CAD build for the part. Positions are in the model's coordinates, mm. Face numbers are marked on the shaded views. A direction names the side the tool comes from. Coordinates: 2 decimals unless noted, no trailing zeros. Write each loop counter-clockwise with the first axis right and the second up, starting at its lowest first coordinate (ties: lowest second). Pieces come first, ordered by that corner, then holes. Notation, with made-up numbers: M -23,34.5 L 30,34.5 A26 cw 30,48.5 Z; hole C -22.5,1.5 d11. An arc over 180 degrees is marked long. Put each result on its own line as item: value. Start each with the question number.
```python
from build123d import *

# Parameters (mm, degrees)
SALIENTE_EXTRUIR1_DEPTH = 22
CROQUIS2_W              = 34
CROQUIS2_H              = 34
SALIENTE_EXTRUIR2_DEPTH = 7
REDONDEO1_R             = 5
CROQUIS3_R              = 3.5
CORTAR_EXTRUIR1_DEPTH   = 5
CROQUIS4_R              = 2
CORTAR_EXTRUIR2_DEPTH   = 5
CROQUIS5_R              = 3.5
CORTAR_EXTRUIR3_DEPTH   = 5
CROQUIS6_R              = 2
CORTAR_EXTRUIR4_DEPTH   = 5
REDONDEO2_R             = 5


with BuildPart() as part:
    # Croquis1 → Saliente-Extruir1 (new body)
    with BuildSketch(Plane(origin=(0, 0, 0), x_dir=(1, 0, 0), z_dir=(0, 1, 0))):
        Polygon((0, 0), (27, 0), (27, 27), (34, 27), (34, -7), (0, -7), align=None)
    extrude(amount=SALIENTE_EXTRUIR1_DEPTH)

    # Croquis2 → Saliente-Extruir2 (add)
    with BuildSketch(Plane(origin=(0, 0, 0), x_dir=(-1, 0, 0), z_dir=(0, -1, 0))):
        with Locations((-17, 10)):
            Rectangle(CROQUIS2_W, CROQUIS2_H)
    extrude(amount=SALIENTE_EXTRUIR2_DEPTH)

    # Redondeo1
    redondeo1_edges = [part.edges().sort_by_distance(p)[0] for p in [
        (34, 7.5, -27),
        (34, 7.5, 7),
        (0, 7.5, 7),
        (34, -7, -10),
        (17, -7, 7),
    ]]
    fillet(redondeo1_edges, radius=REDONDEO1_R)

    # Croquis3 → Cortar-Extruir1 (cut)
    with BuildSketch(Plane(origin=(34, 0, 0), x_dir=(0, 0, -1), z_dir=(1, 0, 0))):
        with Locations((16, 16)):
            Circle(CROQUIS3_R)
    extrude(amount=-CORTAR_EXTRUIR1_DEPTH, mode=Mode.SUBTRACT)

    # Croquis4 → Cortar-Extruir2 (cut)
    with BuildSketch(Plane(origin=(29, 0, 0), x_dir=(0, 0, -1), z_dir=(1, 0, 0))):
        with Locations((16, 16)):
            Circle(CROQUIS4_R)
    extrude(amount=-CORTAR_EXTRUIR2_DEPTH, mode=Mode.SUBTRACT)

    # Croquis5 → Cortar-Extruir3 (cut)
    with BuildSketch(Plane.XY.offset(7)):
        with Locations((11, 16)):
            Circle(CROQUIS5_R)
    extrude(amount=-CORTAR_EXTRUIR3_DEPTH, mode=Mode.SUBTRACT)

    # Croquis6 → Cortar-Extruir4 (cut)
    with BuildSketch(Plane.XY.offset(2)):
        with Locations((11, 16)):
            Circle(CROQUIS6_R)
    extrude(amount=-CORTAR_EXTRUIR4_DEPTH, mode=Mode.SUBTRACT)

    # Redondeo2
    # the kernel refuses this fillet: 5 mm, written as the material it takes off along each edge
    with BuildSketch(Plane(origin=(29, -2, -22), x_dir=(0, -1, 0), z_dir=(0, 0, -1))) as redondeo2_piece_1_section:
        Polygon((0, 0), (REDONDEO2_R, 0), (REDONDEO2_R, -REDONDEO2_R), (0, -REDONDEO2_R), align=None)
    redondeo2_piece_1 = extrude(amount=REDONDEO2_R, mode=Mode.PRIVATE)
    redondeo2_piece_1 = redondeo2_piece_1 - Plane(origin=(29, -2, -22), x_dir=(-0.7071067811865475, 0.7071067811865475, 0), z_dir=(0, 0, -1)) * Sphere(REDONDEO2_R, mode=Mode.PRIVATE)
    add(redondeo2_piece_1, mode=Mode.SUBTRACT)
    with BuildSketch(Plane(origin=(5, -2, 2), x_dir=(0, -1, 0), z_dir=(-1, 0, 0))) as redondeo2_piece_2_section:
        Polygon((0, 0), (REDONDEO2_R, 0), (REDONDEO2_R, REDONDEO2_R), (0, REDONDEO2_R), align=None)
    redondeo2_piece_2 = extrude(amount=REDONDEO2_R, mode=Mode.PRIVATE)
    redondeo2_piece_2 = redondeo2_piece_2 - Plane(origin=(5, -2, 2), x_dir=(0, 0.7071067811865475, -0.7071067811865475), z_dir=(-1, 0, 0)) * Sphere(REDONDEO2_R, mode=Mode.PRIVATE)
    add(redondeo2_piece_2, mode=Mode.SUBTRACT)
    with BuildSketch(Plane(origin=(-12.5, -7, -27), x_dir=(0, 1, 0), z_dir=(1, 0, 0)), Plane(origin=(0, -7, 2), x_dir=(0, 1, 0), z_dir=(0, 0, -1))) as redondeo2_piece_3:
        with BuildLine():
            CenterArc((REDONDEO2_R, REDONDEO2_R), REDONDEO2_R, 180, 90)
            Line((0, REDONDEO2_R), (0, 0))
            Line((0, 0), (REDONDEO2_R, 0))
        make_face()
    extrude(amount=41.5, mode=Mode.SUBTRACT)


solid = part.part
```
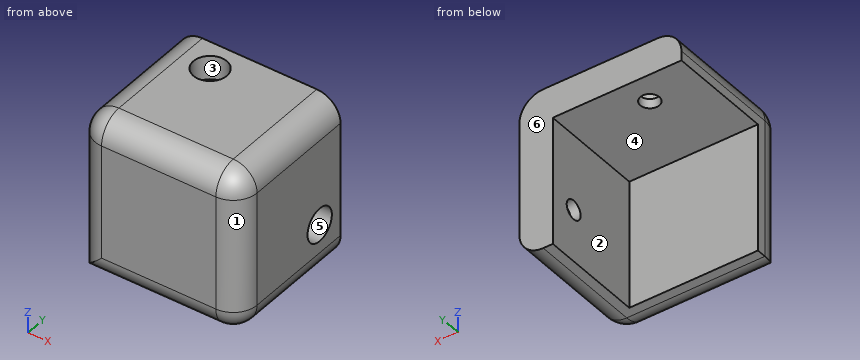
(1) Slice it at D-D, the plane z = -5. Write the cut outline in (x, y), then the cut area to 3 significant figures.
(2) Slice it at A-A, the plane x = 11. Write the cut outline in (y, z).
(3) Which spindle directions (+Z, -Z, +X, -X, +Y, -Y) get a long thin tool onto all of the face, cutting with end or side? Do the marked faces 1, 2 and 3. Say none if no direction does.
(4) Two-plate mould, pull along Z, no slides. Class the marked faces 4, 5 and 6: +Z half, -Z half, draft (parallel to the pull), parting line (faces both ways), or undercut.
(5) Drill centre lines: line 1 (Y direction, x = 28.5, z = -16); line 2 (Z direction, x = 12, y = 6.75); line 3 (X direction, y = -2.25, z = -1). Where is each one in solid material? Low to high. Write a range as [from, to].
(6) Slice it at B-B, the plane z = -16. Write the cut outline in (x, y), then the cut area to 3 significant figures.
(7) Drop flat-ended pins along their axis: pin 1 (12 mm diameter, centred on y = 14.5, z = -11, fed in from -X); pin 2 (3 mm diameter, centred on y = 16, z = -16, fed in from +X); pin 3 (11 mm diameter, centred on x = 11, y = 16, fed in from -Z). Give the stop position or say it passes through.
(8) Slice it at C-C, the plane y = 14.75. Write the cut outline in (x, z), then the cut area to 3 significant figures.
Result set:
1. outline: M 0,-2 A5 ccw 5,-7 L 29,-7 A5 ccw 34,-2 L 34,22 L 27,22 L 27,0 L 0,0 Z
1. area: 381 mm^2
2. outline: M -7,-22 A5 ccw -2,-27 L 0,-27 L 0,0 L 14,0 L 14,2 L 12.5,2 L 12.5,7 L -2,7 A5 ccw -7,2 Z; M 18,0 L 22,0 L 22,7 L 19.5,7 L 19.5,2 L 18,2 Z
3. face 1: +Z, -Z, +X, -Y
3. face 2: -Z, -X, +Y
3. face 3: +Z
4. face 4: -Z half
4. face 5: undercut
4. face 6: draft
5. line 1: y = [-7, 14], [18, 22]
5. line 2: z = [0, 7]
5. line 3: x = [0.01, 33.99]
6. outline: M 0,-2 A5 ccw 5,-7 L 29,-7 A5 ccw 34,-2 L 34,12.5 L 29,12.5 L 29,14 L 27,14 L 27,0 L 0,0 Z; M 27,18 L 29,18 L 29,19.5 L 34,19.5 L 34,22 L 27,22 Z
6. area: 338 mm^2
7. pin 1: stops at x = 27
7. pin 2: passes through
7. pin 3: stops at z = 0
8. outline: M 0,0 L 9.44,0 L 9.44,2 L 7.73,2 L 7.73,7 L 5,7 A5 ccw 0,2 Z; M 12.56,0 L 27,0 L 27,-14.44 L 29,-14.44 L 29,-12.73 L 34,-12.73 L 34,2 A5 ccw 29,7 L 14.27,7 L 14.27,2 L 12.56,2 Z; M 27,-27 L 29,-27 A5 ccw 34,-22 L 34,-19.27 L 29,-19.27 L 29,-17.56 L 27,-17.56 Z
8. area: 333 mm^2
